```python
from build123d import *

# Parameters (mm, degrees)
ESQUISSE3_R             = 1.625
ESQUISSE3_R_2           = 6
BOSS_EXTRU_1_DEPTH      = 3.5
ESQUISSE4_R             = 14.5
ESQUISSE4_R_2           = 7.5
BOSS_EXTRU_2_DEPTH      = 9.525
CONG_3_R                = 6
ENL_V_MAT_EXTRU_1_DEPTH = 37.971588497
ENL_V_MAT_EXTRU_2_DEPTH = 37.971588497


with BuildPart() as part:
    # Esquisse3 → Boss.-Extru.1 (new body)
    with BuildSketch(Plane.XY):
        Polygon((0, -31.754264805), (-27.5, 15.877132403), (27.5, 15.877132403), align=None)
        with Locations((-17.5, 10.103629711)):
            Circle(ESQUISSE3_R, mode=Mode.SUBTRACT)
        with Locations((17.5, 10.103629711)):
            Circle(ESQUISSE3_R, mode=Mode.SUBTRACT)
        with Locations((0, -20.207259422)):
            Circle(ESQUISSE3_R, mode=Mode.SUBTRACT)
        Circle(ESQUISSE3_R_2, mode=Mode.SUBTRACT)
    extrude(amount=BOSS_EXTRU_1_DEPTH)

    # Esquisse4 → Boss.-Extru.2 (add)
    with BuildSketch(Plane.XY.offset(3.5)):
        Circle(ESQUISSE4_R)
        Circle(ESQUISSE4_R_2, mode=Mode.SUBTRACT)
    extrude(amount=BOSS_EXTRU_2_DEPTH)

    # Congé3
    cong_3_edges = [part.edges().sort_by_distance(p)[0] for p in [
        (0, -31.754264805, 1.75),
        (-27.5, 15.877132403, 1.75),
        (27.5, 15.877132403, 1.75),
    ]]
    fillet(cong_3_edges, radius=CONG_3_R)

    # Esquisse5 → Enlèv. mat.-Extru.1 (cut, through all)
    with BuildSketch(Plane.XY.offset(13.025)):
        with BuildLine():
            ThreePointArc((-7.238095238, 6.153046183), (0, 9.5), (7.238095238, 6.153046183))
            ThreePointArc((7.238095238, 6.153046183), (8.647689072, 6.038830492), (8.761904762, 7.448424326))
            ThreePointArc((8.761904762, 7.448424326), (0, 11.5), (-8.761904762, 7.448424326))
            ThreePointArc((-8.761904762, 7.448424326), (-8.647689072, 6.038830492), (-7.238095238, 6.153046183))
        make_face()
    extrude(amount=-ENL_V_MAT_EXTRU_1_DEPTH, mode=Mode.SUBTRACT)

    # Esquisse6 → Enlèv. mat.-Extru.2 (cut, through all)
    with BuildSketch(Plane.XY.offset(13.025)):
        with BuildLine():
            ThreePointArc((-2.322580645, 5.532234553), (-1.386431589, 7.823222319), (-3.677419355, 8.759371375))
            ThreePointArc((-3.677419355, 8.759371375), (0, 9.5), (3.677419355, 8.759371375))
            ThreePointArc((3.677419355, 8.759371375), (1.386431589, 7.823222319), (2.322580645, 5.532234553))
            ThreePointArc((2.322580645, 5.532234553), (0, 6), (-2.322580645, 5.532234553))
        make_face()
    extrude(amount=-ENL_V_MAT_EXTRU_2_DEPTH, mode=Mode.SUBTRACT)


solid = part.part
```
Could you check a few things on this model? Use its own coordinates, in mm. A direction names the side the tool comes from. Round coordinates to 2 decimals unless told otherwise and drop trailing zeros. Loops run counter-clockwise (first coordinate to the right, second up) from the corner with the lowest first, then second, coordinate; pieces in that order, holes last. Notation, with made-up numbers: M 42,-15.5 L 94,-15.5 A23 ccw 94,19.5 Z; hole C 85.5,32.5 d6. An arc over 180 degrees is marked long. Write item = value, one per line.
1. I want a section at B-B, the plane z = 12. Write out the boundary of the cut face in (x, y), and give its area (3 significant figures).
Results below:
outline = C 0,0 d29; hole M -8.76,7.45 A1 ccw -7.24,6.15 A9.5 cw -3.68,8.76 A1.75 cw -1.27,7.39 A7.5 ccw long 1.27,7.39 A1.75 cw 3.68,8.76 A9.5 cw 7.24,6.15 A1 ccw 8.76,7.45 A11.5 ccw Z
area = 437 mm²
2. Will these pins go through, and if not, where does the flat tip stop? P1, Ø12, axis at x = 3, y = 1, coming from the +Z side (3 decimals); P2, Ø6, axis at x = -8, z = 9, coming from the -Y side; P3, Ø5, axis at x = 3, z = 2, coming from the -Y side; P4, Ø1.9, axis at x = 0, y = -20.21, coming from the +Z side.
Results below:
P1 = 13.025
P2 = -13.61
P3 = -25.73
P4 = through
3. I want a section at C-C, the plane x = -3. Write out the boundary of the cut face in (y, z) (3 decimals).
Results below:
outline = M -24.95,0 L -5.196,0 L -5.196,3.5 L -6.874,3.5 L -6.874,13.025 L -14.186,13.025 L -14.186,3.5 L -24.95,3.5 Z; M 5.196,0 L 8.896,0 L 8.896,13.025 L 6.874,13.025 L 6.874,3.5 L 5.196,3.5 Z; M 11.102,0 L 15.877,0 L 15.877,3.5 L 14.186,3.5 L 14.186,13.025 L 11.102,13.025 Z
4. I want a section at D-D, the plane z = 1.75. Write out the boundary of the cut face in (x, y) (3 decimals), and give its area (3 significant figures).
Results below:
outline = M -22.304,6.877 L -5.196,-22.754 A6 ccw 5.196,-22.754 L 22.304,6.877 A6 ccw 17.108,15.877 L -17.108,15.877 A6 ccw Z; hole C -17.5,10.104 d3.25; hole M -8.762,7.448 A1 ccw -7.238,6.153 A9.5 cw -3.677,8.759 A1.75 cw -2.323,5.532 A6 ccw long 2.323,5.532 A1.75 cw 3.677,8.759 A9.5 cw 7.238,6.153 A1 ccw 8.762,7.448 A11.5 ccw Z; hole C 0,-20.207 d3.25; hole C 17.5,10.104 d3.25
area = 1,050 mm²
5. I need wall thicknesses on probe 1 along Z at (x, y) = (-6, -4); probe 2 along Y at (x, z) = (-17.5, 1.85); probe 3 along X at (y, z) = (4.5, 7). Which ranges of each line are inside material? Lowest first, please.
Results below:
probe_1 = 0 to 3.5
probe_2 = -1.44 to 8.48, 11.73 to 15.86
probe_3 = -13.78 to -6, 6 to 13.78
6. I want a section at A-A, the plane x = -18.5. Write out the boundary of the cut face in (y, z), and give its area (3 significant figures).
Results below:
outline = M 0.29,0 L 8.82,0 L 8.82,3.5 L 0.29,3.5 Z; M 11.38,0 L 15.71,0 L 15.71,3.5 L 11.38,3.5 Z
area = 45.0 mm²
7. Thinking about a two-plate mould opening in X: for faces 4 (the face through (-8.66, 6.05, 6.6)), 5 (the face through (-13.63, -8.15, 1.73)), 6 (the face through (13.87, -7.73, 1.73)), 7 (the face through (-5, -5, 0)), which applies, +X half, -X half, draft (parallel to the pull), parting line (faces both ways), or undercut?
Results below:
face_4 = undercut
face_5 = -X half
face_6 = +X half
face_7 = draft
8. Which directions (+Z, -Z, +X, -X, +Y, -Y) give clear straight access to the entire face, cutting with the end or side of a thin tool? Please do faces 1 (the face through (22.347, 12.801, 1.774)), 2 (the face through (-0.312, -7.494, 8.196)), 3 (the face through (0.1, 11.5, 6.6)).
Results below:
face_1 = +Z, -Z, +X
face_2 = +Z
face_3 = +Z, -Z
